from build123d import *

# Parameters (mm, degrees)
F0_W     = 3.175
F0_H     = 8.89
F1_DEPTH = 3.175
F2_R     = 1.5875
F3_DEPTH = 3.176


# Not quite as in the source:
# - a feature names something its author has since deleted; it is built from what else it names


with BuildPart() as f1:
    # F0 (on Front) → F1 (new body)
    with BuildSketch(Plane.XZ):
        Polygon((9.525, 11.43), (9.525, 38.1), (-6.35, 38.1), (-6.35, 29.21), (-6.35, 20.32), (-6.35, 11.43), align=None)
        with Locations((-7.9375, 33.655)):
            Rectangle(F0_W, F0_H)
        with Locations((-7.9375, 15.875)):
            Rectangle(F0_W, F0_H)
    extrude(amount=F1_DEPTH)

    # F2 (on face) → F3 (cut, through all)
    with BuildSketch(Plane.XZ.offset(3.175)):
        with Locations((1.5875, 24.6701687584)):
            Circle(F2_R)
    extrude(amount=-F3_DEPTH, mode=Mode.SUBTRACT)


solid = f1.part
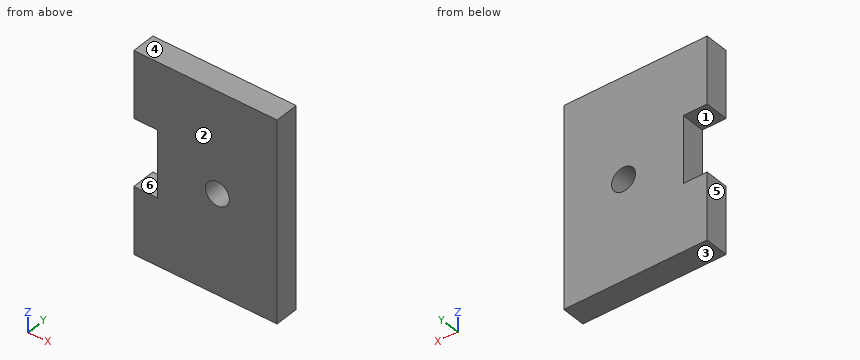
Geometry: final body of the model. Coordinates: model frame, mm. Face numbers are marked on the shaded views. A direction names the side the tool comes from. Coordinates: 2 decimals unless noted, no trailing zeros. Loops run counter-clockwise (first coordinate to the right, second up) from the corner with the lowest first, then second, coordinate; pieces in that order, holes last. Notation, with made-up numbers: M 4.5,69 L 45.5,69 A21 cw 45.5,102 Z; hole C 65.25,42.25 d11. An arc over 180 degrees is marked long. One line per item, written item: value. Start each with the question number.
1) Reachability of the marked faces 5 and 6 from +Z, -Z, +X, -X, +Y, -Y: full face, straight path, thin tool, end or side. Return the list, or none.
2) Material intervals for L1, parallel to Z at x = -7, y = -0.3; L2, parallel to X at y = -2.2, z = 22.5 (3 decimals); L3, parallel to Z at x = 0.75, y = -2.95, sorted ascending. Write a range as from..to.
3) Pin query (flat end, axial travel): P1, Ø1, axis at y = -1.5, z = 23, coming from the -X side. Return the tip coordinate at first contact, or that it passes through.
4) Cut plane C-C (z = 28). Return loops of the section in (x, y) (3 decimals), then the cut area to 3 significant figures.
5) Draft query along Z for the marked faces 1, 2, 3 and 4. Return one class per face: released by +Z, released by -Z, zero draft, split by the parting line, or undercut.
6) Cut plane A-A (z = 24.25). Return loops of the section in (x, y) (3 decimals).
Evaluation:
1. face 5: +Z, -Z, -X, +Y, -Y
1. face 6: -X, +Y, -Y
2. L1: 11.43..20.32, 29.21..38.1
2. L2: -6.35..9.525
2. L3: 11.43..23.32, 26.02..38.1
3. P1: x = -6.35
4. outline: M -6.35,-3.175 L 9.525,-3.175 L 9.525,0 L -6.35,0 Z
4. area: 50.4 mm^2
5. face 1: undercut
5. face 2: zero draft
5. face 3: released by -Z
5. face 4: released by +Z
6. outline: M -6.35,-3.175 L 0.057,-3.175 L 0.057,0 L -6.35,0 Z; M 3.118,-3.175 L 9.525,-3.175 L 9.525,0 L 3.118,0 Z
